Can you work these out from the model? Positions are in its coordinate system, mm. Give positions to 0.01 mm unless a question says otherwise; leave off trailing zeros. Loops run counter-clockwise (first coordinate to the right, second up) from the corner with the lowest first, then second, coordinate; pieces in that order, holes last. Notation, with made-up numbers: (19.25, 87.5) -> (39.25, 87.5) arc R27 ccw to (39.25, 123.5) -> close; hole circle Ø5 at (82.25, 32). An arc over 180 degrees is marked (long way). One line per question, with ' | ' between items.
Autodesk Inventor part; units mm, degrees
ref_plane "YZ Plane" through (0, 0, 0) normal (1, 0, 0) x (0, 1, 0)
ref_plane "XZ Plane" through (0, 0, 0) normal (0, 1, 0) x (-1, 0, 0)
ref_plane "XY Plane" through (0, 0, 0) normal (0, 0, 1) x (1, 0, 0)
sketch "Sketch1" plane through (0, 0, 0) normal (0, 0, 1) x (1, 0, 0)
  line L0 (-125.8778, 76.6863) -> (128.1222, 76.6863)
  line L1 (128.1222, 76.6863) -> (128.1222, -63.0137)
  line L2 (128.1222, -63.0137) -> (-125.8778, -63.0137)
  line L3 (-125.8778, -63.0137) -> (-125.8778, 76.6863)
  line L4 (-125.8778, -63.0137) -> (-94.1278, -63.0137)
  line L5 (-94.1278, -63.0137) -> (-94.1278, -43.9637)
  line L6 (-94.1278, -43.9637) -> (-36.9778, -43.9637)
  line L7 (-36.9778, -43.9637) -> (-36.9778, -63.0137)
  line L8 (128.1222, -63.0137) -> (58.2722, -63.0137)
  line L9 (58.2722, -63.0137) -> (58.2722, -50.3137)
  line L10 (58.2722, -50.3137) -> (39.2222, -50.3137)
  line L11 (39.2222, -50.3137) -> (39.2222, -63.0137)
  line L12 (-125.8778, 76.6863) -> (-113.1778, 76.6863)
  line L13 (-113.1778, 76.6863) -> (-113.1778, 63.9863)
  circle A0 centre (-113.1778, 63.9863) radius 2.54
  line L14 (-113.1778, 63.9863) -> (1.1222, 63.9863)
  circle A1 centre (1.1222, 63.9863) radius 2.54
  line L15 (1.1222, 63.9863) -> (115.4222, 63.9863)
  circle A2 centre (115.4222, 63.9863) radius 2.54
  line L16 (-125.8778, -63.0137) -> (-113.1778, -63.0137)
  line L17 (-113.1778, -63.0137) -> (-113.1778, -50.3137)
  circle A3 centre (-113.1778, -50.3137) radius 2.54
  line L18 (128.1222, -63.0137) -> (128.1222, -50.3137)
  line L19 (128.1222, -50.3137) -> (115.4222, -50.3137)
  circle A4 centre (115.4222, -50.3137) radius 2.54
  point P0 (0, 0)
  dimension "d0" = 254
  dimension "d1" = 139.7
  dimension "d6" = 31.75
  dimension "d7" = 19.05
  dimension "d8" = 57.15
  dimension "d9" = 69.85
  dimension "d10" = 12.7
  dimension "d11" = 19.05
  dimension "d14" = 12.7
  dimension "d15" = 12.7
  dimension "d16" = 5.08
  dimension "d17" = 114.3
  dimension "d18" = 5.08
  dimension "d19" = 114.3
  dimension "d20" = 5.08
  dimension "d21" = 12.7
  dimension "d22" = 12.7
  dimension "d23" = 5.08
  dimension "d24" = 12.7
  dimension "d25" = 12.7
  dimension "d26" = 5.08
extrude "Extrusion4" add sketch "Sketch1" along normal blind 0.7937 contours L0 L1 L2 L9 L10 L11 L7 L6 L5 L3
properties part number "Top Intake Poly (Sponsor Panel)"
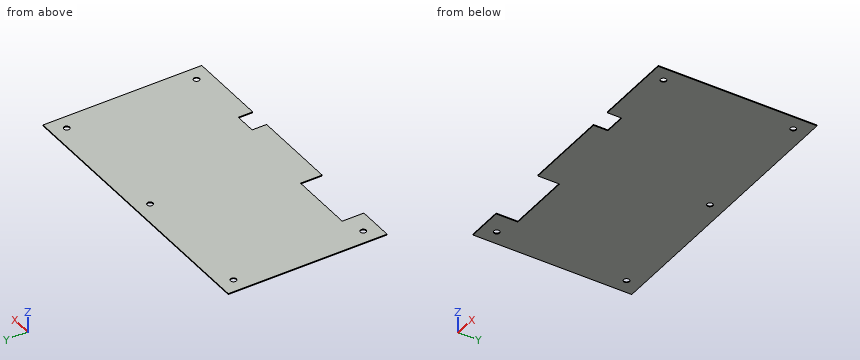
Q1. If we section it at A-A (z = 0.65): Write out the boundary of the cut face in (x, y).
Entries:
outline: (-125.88, -63.01) -> (-94.13, -63.01) -> (-94.13, -43.96) -> (-36.98, -43.96) -> (-36.98, -63.01) -> (39.22, -63.01) -> (39.22, -50.31) -> (58.27, -50.31) -> (58.27, -63.01) -> (128.12, -63.01) -> (128.12, 76.69) -> (-125.88, 76.69) -> close; hole circle Ø5.08 at (-113.18, -50.31); hole circle Ø5.08 at (-113.18, 63.99); hole circle Ø5.08 at (1.12, 63.99); hole circle Ø5.08 at (115.42, -50.31); hole circle Ø5.08 at (115.42, 63.99)
Q2. If I drill on probe 1 along X at (y, z) = (-46, 0.6); probe 2 along Y at (x, z) = (48, 0.45); probe 3 along Y at (x, z) = (-37.5, 0.25), over which ranges is the centre line in solid material (lowest first)? Write a range as from..to.
Entries:
probe 1: -125.88..-94.13, -36.98..128.12 | probe 2: -50.31..76.69 | probe 3: -43.96..76.69
Q3. For pin 1 Ø4.5 at (x, y) = (-113.18, -50.31) entering from -Z, with a flat end and sliding along its axis, tell me the tip position at first contact or that it passes through.
Entries:
pin 1: through
Q4. If we section it at B-B (x = -42): Write out the boundary of the cut face in (y, z).
Entries:
outline: (-43.96, 0) -> (76.69, 0) -> (76.69, 0.79) -> (-43.96, 0.79) -> close
